```python
from build123d import *
from build123d.topology import SkipClean

# Parameters (mm, degrees)
SKETCH2_R           = 5.1
BOSS_EXTRUDE1_DEPTH = 1
SKETCH3_R           = 5.1
SKETCH3_R_2         = 4.3
BOSS_EXTRUDE2_DEPTH = 12
CUT_EXTRUDE2_DEPTH  = 1
SKETCH7_R           = 7.5
SKETCH7_R_2         = 5.1
BOSS_EXTRUDE4_DEPTH = 2


with BuildPart() as part:
    # Sketch2 → Boss-Extrude1 (new body)
    with BuildSketch(Plane(origin=(0, 0, 0), x_dir=(1, 0, 0), z_dir=(0, 1, 0))):
        with Locations(Location((0, 0, 0), (0, 0, 270))):
            Circle(SKETCH2_R)
    extrude(amount=BOSS_EXTRUDE1_DEPTH)

    # Sketch3 → Boss-Extrude2 (add)
    with BuildSketch(Plane(origin=(0, 1, 0), x_dir=(1, 0, 0), z_dir=(0, 1, 0))):
        with Locations(Location((0, 0, 0), (0, 0, 270))):
            Circle(SKETCH3_R)
        with Locations(Location((0, 0, 0), (0, 0, 270))):
            Circle(SKETCH3_R_2, mode=Mode.SUBTRACT)
    extrude(amount=BOSS_EXTRUDE2_DEPTH)

    # Sketch6 → Cut-Extrude2 (cut)
    with BuildSketch(Plane(origin=(0, 1, 0), x_dir=(1, 0, 0), z_dir=(0, 1, 0))):
        with BuildLine():
            ThreePointArc((-1.767766953, 1.767766953), (-2.165063509, 1.25), (-2.414814566, 0.647047613))
            Line((-2.414814566, 0.647047613), (-3.187555227, 0.854102849))
            ThreePointArc((-3.187555227, 0.854102849), (-2.857883832, 1.65), (-2.333452378, 2.333452378))
            Line((-2.333452378, 2.333452378), (-1.767766953, 1.767766953))
        make_face()
        with BuildLine():
            ThreePointArc((2.414814566, 0.647047613), (2.165063509, 1.25), (1.767766953, 1.767766953))
            Line((1.767766953, 1.767766953), (2.333452378, 2.333452378))
            ThreePointArc((2.333452378, 2.333452378), (2.857883832, 1.65), (3.187555227, 0.854102849))
            Line((3.187555227, 0.854102849), (2.414814566, 0.647047613))
        make_face()
        with BuildLine():
            ThreePointArc((1.767766953, -1.767766953), (2.165063509, -1.25), (2.414814566, -0.647047613))
            Line((2.414814566, -0.647047613), (3.187555227, -0.854102849))
            ThreePointArc((3.187555227, -0.854102849), (2.857883832, -1.65), (2.333452378, -2.333452378))
            Line((2.333452378, -2.333452378), (1.767766953, -1.767766953))
        make_face()
        with BuildLine():
            ThreePointArc((-0.647047613, -2.414814566), (0, -2.5), (0.647047613, -2.414814566))
            Line((0.647047613, -2.414814566), (0.854102849, -3.187555227))
            ThreePointArc((0.854102849, -3.187555227), (0, -3.3), (-0.854102849, -3.187555227))
            Line((-0.854102849, -3.187555227), (-0.647047613, -2.414814566))
        make_face()
        with BuildLine():
            ThreePointArc((-2.414814566, -0.647047613), (-2.165063509, -1.25), (-1.767766953, -1.767766953))
            Line((-1.767766953, -1.767766953), (-2.333452378, -2.333452378))
            ThreePointArc((-2.333452378, -2.333452378), (-2.857883832, -1.65), (-3.187555227, -0.854102849))
            Line((-3.187555227, -0.854102849), (-2.414814566, -0.647047613))
        make_face()
        with BuildLine():
            ThreePointArc((0.647047613, 2.414814566), (0, 2.5), (-0.647047613, 2.414814566))
            Line((-0.647047613, 2.414814566), (-0.854102849, 3.187555227))
            ThreePointArc((-0.854102849, 3.187555227), (0, 3.3), (0.854102849, 3.187555227))
            Line((0.854102849, 3.187555227), (0.647047613, 2.414814566))
        make_face()
    extrude(amount=-CUT_EXTRUDE2_DEPTH, mode=Mode.SUBTRACT)

    # Sketch7 → Boss-Extrude4 (add)
    with BuildSketch(Plane(origin=(0, 6, 0), x_dir=(1, 0, 0), z_dir=(0, 1, 0))):
        with Locations(Location((0, 0, 0), (0, 0, 270))):
            Circle(SKETCH7_R)
        with Locations(Location((0, 0, 0), (0, 0, 270))):
            Circle(SKETCH7_R_2, mode=Mode.SUBTRACT)
    extrude(amount=BOSS_EXTRUDE4_DEPTH)

    # Sketch10 → Revolve1 (revolve)
    with SkipClean():  # the faces are left unmerged after this step: merging them gives an invalid solid
        with BuildSketch(Plane(origin=(0, 0, 0), x_dir=(0, 0, -1), z_dir=(1, 0, 0)), mode=Mode.PRIVATE) as revolve1_sk:
            with BuildLine():
                ThreePointArc((1.5, -2.4), (0.764852927, -2.175735365), (0, -2.1))
                Line((0, -2.1), (0, -6))
                Line((0, -6), (0, -9.9))
                ThreePointArc((0, -9.9), (2.757716447, -8.757716447), (3.9, -6))
                ThreePointArc((3.9, -6), (3.244996148, -3.836669235), (1.5, -2.4))
            make_face()
            with BuildLine():
                Line((0, -6), (0, -2.1))
                ThreePointArc((0, -2.1), (-0.764852927, -2.175735365), (-1.5, -2.4))
                ThreePointArc((-1.5, -2.4), (-3.824264635, -6.764852927), (0, -9.9))
                Line((0, -9.9), (0, -6))
            make_face()
            with BuildLine():
                Line((0, -2.1), (0, 0))
                Line((0, 0), (-1.5, 0))
                Line((-1.5, 0), (-1.5, -2.4))
                ThreePointArc((-1.5, -2.4), (-0.764852927, -2.175735365), (0, -2.1))
            make_face()
        revolve(revolve1_sk.sketch.rotate(Axis((0, -2.1, 0), (0, -1, 0)), 180), axis=Axis((0, -2.1, 0), (0, -1, 0)))


solid = part.part
```
The listing builds one solid part. Answer for the finished solid, in the listing's coordinates (mm). A direction names the side the tool comes from. Give positions to 0.01 mm unless a question says otherwise; leave off trailing zeros. Write each loop counter-clockwise with the first axis right and the second up, starting at its lowest first coordinate (ties: lowest second). Pieces come first, ordered by that corner, then holes. Notation, with made-up numbers: M -17,81.25 L 7,81.25 A31 ccw 7,120.25 Z; hole C 16.25,-10 d6. An arc over 180 degrees is marked long. Write each question's results on one line, items separated by ' | '.
Q1. Section C-C, the plane y = 10 is taken. Write down the section's boundary in (x, z).
Output values:
outline: C 0,0 d10.2; hole C 0,0 d8.6
Q2. Flat-ended cylindrical pins translate along their axes: P1, Ø7, axis at x = -0.5, z = 0.5, coming from the +Y side; P2, Ø6, axis at x = -4, y = -4, coming from the -Z side; P3, Ø3, axis at x = -2, z = 0, coming from the -Y side; P4, Ø6, axis at x = 0, z = 6, coming from the +Y side. Find the tip coordinate at first contact, or state that the pin passes through.
Output values:
P1: y = 1 | P2: z = -3.61 | P3: y = -9.87 | P4: y = 13
Q3. Section A-A, the plane x = 0 is taken. Write down the section's boundary in (y, z).
Output values:
outline: M -2.4,-1.5 L 0,-1.5 L 0,-2.5 L 1,-2.5 L 1,2.5 L 0,2.5 L 0,1.5 L -2.4,1.5 A3.9 ccw long Z; M 0,-5.1 L 6,-5.1 L 6,-7.5 L 8,-7.5 L 8,-5.1 L 13,-5.1 L 13,-4.3 L 1,-4.3 L 1,-3.3 L 0,-3.3 Z; M 0,3.3 L 1,3.3 L 1,4.3 L 13,4.3 L 13,5.1 L 8,5.1 L 8,7.5 L 6,7.5 L 6,5.1 L 0,5.1 Z
Q4. For a pull along X with two mould halves and no side action, classify faces 4 (the flat face through (-5, 6, 2)), 5 (the cylindrical face through (1.532, 10.465, 4.864)), 6 (the cylindrical face through (-2.85, 0.51, 1.66)) as released by +X, released by -X, zero draft, split by the parting line, or undercut.
Output values:
face 4: zero draft | face 5: split by the parting line | face 6: undercut
Q5. Consider L1, parallel to X at y = 4.25, z = 0; L2, parallel to Z at x = -2, y = 0.5; L3, parallel to X at y = 7.5, z = 0. Determine where each line is inside the solid, lowest interval first. Write a range as from..to.
Output values:
L1: -5.1..-4.3, 4.3..5.1 | L2: -4.69..-2, -1.5..1.5, 2..4.69 | L3: -7.5..-4.3, 4.3..7.5
Q6. Section B-B, the plane z = 0 is taken. Write down the section's boundary in (x, y).
Output values:
outline: M -7.5,6 L -5.1,6 L -5.1,0 L -1.5,0 L -1.5,-2.4 A3.9 ccw long 1.5,-2.4 L 1.5,0 L 5.1,0 L 5.1,6 L 7.5,6 L 7.5,8 L 5.1,8 L 5.1,13 L 4.3,13 L 4.3,1 L -4.3,1 L -4.3,13 L -5.1,13 L -5.1,8 L -7.5,8 Z
Q7. A tool of negligible diameter and unlimited length cuts with its end or side. For faces 1 (the cylindrical face through (0.45, -1.22, -1.43)), 2 (the cylindrical face through (2.16, 0.51, 1.26)), 3 (the flat face through (-4, 13, -2)), from which of +Z, -Z, +X, -X, +Y, -Y can it reach the whole face along a straight path? Write none if from no direction.
Output values:
face 1: none | face 2: +Y | face 3: +Z, -Z, +X, -X, +Y
Q8. Section D-D, the plane y = -4 is taken. Write down the section's boundary in (x, z).
Output values:
outline: C 0,0 d6.7
